```python
from build123d import *

# Parameters (mm, degrees)
BOSS_EXTRUDE1_DEPTH = 10
BOSS_EXTRUDE3_DEPTH = 10
FILLET3_R           = 1.5


with BuildPart() as part:
    # Sketch1 → Boss-Extrude1 (new body)
    with BuildSketch(Plane.XY):
        Polygon((-12.5, -2), (12.5, -2), (12.5, -47.6), (15, -47.6), (15, -2), (15, 2), (-15, 2), (-15, -2), (-15, -47.6), (-12.5, -47.6), align=None)
    extrude(amount=BOSS_EXTRUDE1_DEPTH)

    # Sketch2 → Boss-Extrude3 (add)
    with BuildSketch(Plane.XY.offset(10)):
        Polygon((18, -44.6), (15, -47.6), (15, -44.6), align=None)
        Polygon((-15, -47.6), (-15, -44.6), (-18, -44.6), align=None)
    extrude(amount=-BOSS_EXTRUDE3_DEPTH)

    # Fillet3
    fillet3_edges = [part.edges().sort_by_distance(p)[0] for p in [
        (12.5, -24.8, 0),
        (0, -2, 0),
        (-12.5, -24.8, 0),
        (-12.5, -24.8, 10),
        (0, -2, 10),
        (12.5, -24.8, 10),
    ]]
    fillet(fillet3_edges, radius=FILLET3_R)


solid = part.part
```
For this review, take the finished solid that the model builds, in its own axes (mm). A direction names the side the tool comes from. Coordinates: 2 decimals unless noted, no trailing zeros. Write each loop counter-clockwise with the first axis right and the second up, starting at its lowest first coordinate (ties: lowest second). Pieces come first, ordered by that corner, then holes. Notation, with made-up numbers: (52.25, 55.25) - (93.25, 55.25) arc R17 ccw to (93.25, 74.25) - close; hole circle Ø11 at (9, 50.5). An arc over 180 degrees is marked (long way). Put each result on its own line as item: value.
1. Add section A-A, the plane y = -42. Give the boundary of the cut face in (x, z), then the cut area to 3 significant figures.
Values found:
outline: (-15, 0) - (-14, 0) arc R1.5 ccw to (-12.5, 1.5) - (-12.5, 8.5) arc R1.5 ccw to (-14, 10) - (-15, 10) - close; (12.5, 1.5) arc R1.5 ccw to (14, 0) - (15, 0) - (15, 10) - (14, 10) arc R1.5 ccw to (12.5, 8.5) - close
area: 48.1 mm²
2. Add section C-C, the plane y = -1.5. Give the boundary of the cut face in (x, z), then the cut area to 3 significant figures.
Values found:
outline: (-15, 0) - (-14, 0) arc R1.5 ccw to (-13, 0.38) - (13, 0.38) arc R1.5 ccw to (14, 0) - (15, 0) - (15, 10) - (14, 10) arc R1.5 ccw to (13, 9.62) - (-13, 9.62) arc R1.5 ccw to (-14, 10) - (-15, 10) - close
area: 280 mm²
3. Add section B-B, the plane z = 3.5. Give the boundary of the cut face in (x, y).
Values found:
outline: (-18, -44.6) - (-15, -47.6) - (-12.5, -47.6) - (-12.5, -2) - (12.5, -2) - (12.5, -47.6) - (15, -47.6) - (18, -44.6) - (15, -44.6) - (15, 2) - (-15, 2) - (-15, -44.6) - close
4. Add section D-D, the plane x = 4.5. Give the boundary of the cut face in (y, z), then the cut area to 3 significant figures.
Values found:
outline: (-2, 1.5) arc R1.5 ccw to (-0.5, 0) - (2, 0) - (2, 10) - (-0.5, 10) arc R1.5 ccw to (-2, 8.5) - close
area: 39.0 mm²
5. For pin 1 (4 mm diameter, centred on y = -10, z = 2, fed in from +X); pin 2 (5 mm diameter, centred on y = -22, z = 7, fed in from -X); pin 3 (0.9 mm diameter, centred on x = 16, z = 4, fed in from +Y), all flat-tipped, find the tip position at first contact; note any pin that passes through.
Values found:
pin 1: x = 15
pin 2: x = -15
pin 3: y = -44.6
6. Mouldability with a two-part tool opening along X and no side actions: class faces 1 (the flat face through (-15, -21, 5)), 2 (the flat face through (16, -44.6, 5)), 3 (the flat face through (0, -2, 5)), 4 (the flat face through (15, -22, 5)) as released by +X, released by -X, zero draft, split by the parting line, or undercut.
Values found:
face 1: released by -X
face 2: zero draft
face 3: undercut
face 4: released by +X
7. Wall thickness on probe 1 along X at (y, z) = (-2.5, 7); probe 2 along Y at (x, z) = (-10.5, 5.5); probe 3 along X at (y, z) = (-27.5, 0.5): over which ranges is each line inside the solid? List them lowest first.
Values found:
probe 1: -15 to -12.5, 12.5 to 15
probe 2: -2 to 2
probe 3: -15 to -12.88, 12.88 to 15
8. Machinability: for faces 5 (the flat face through (-16, -44.6, 5)), 6 (the cylindrical face through (-12.95, -23.72, 9.57)), 7 (the cylindrical face through (12.95, -24.38, 0.43)), 8 (the flat face through (16.5, -46.1, 5.1)), 9 (the flat face through (12.5, -24, 5)), which of the approach directions +Z, -Z, +X, -X, +Y, -Y give a long, thin tool a straight path to every point of the face, cutting with its end or side? Answer none if there is none.
Values found:
face 5: +Z, -Z, -X, +Y
face 6: +Z, -Y
face 7: -Z, -Y
face 8: +Z, -Z, +X, -Y
face 9: +Z, -Z, -Y
